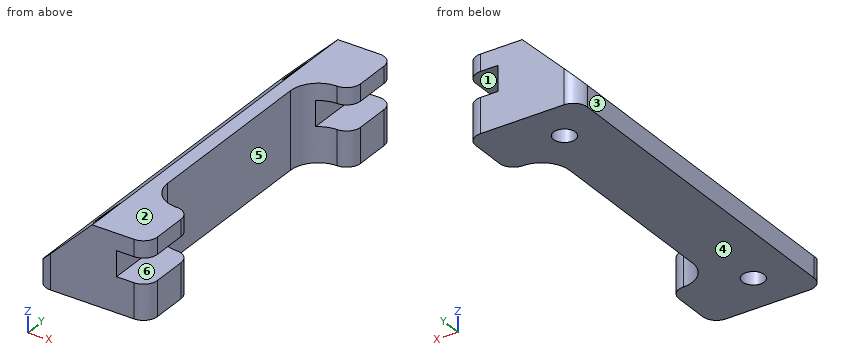
Autodesk Inventor part; units mm, degrees
ref_plane "YZ Plane" through (0, 0, 0) normal (1, 0, 0) x (0, 1, 0)
ref_plane "XZ Plane" through (0, 0, 0) normal (0, 1, 0) x (-1, 0, 0)
ref_plane "XY Plane" through (0, 0, 0) normal (0, 0, 1) x (1, 0, 0)
sketch "Sketch1" plane through (0, 0, 0) normal (0, 0, 1) x (1, 0, 0)
  line L0 (-4, 13) -> (-4, -13)
  line L1 (-4, -13) -> (4, -13)
  line L2 (4, -13) -> (4, 13)
  line L3 (4, 13) -> (-4, 13)
  line L4 (-1, -10) -> (-1, 10) construction
  circle A0 centre (-1, 10) radius 3 construction
  point P0 (0, 0)
  point P1 (0, 13)
  point P2 (-4, 0)
  point P3 (-1, 0)
  dimension "d0" = 26
  dimension "d2" = 20
  dimension "d5" = 5
extrude "Extrusion1" add sketch "Sketch1" along normal mid plane 5.5
sketch "Sketch2" plane through (0, 0, 2.75) normal (0, 0, 1) x (1, 0, 0)
  point P0 (0, 0)
  point P1 (-1, 10)
  point P2 (-1, -10)
hole "Hole1" at (-1, 10, 2.75) at (-1, -10, 2.75) direction (0, 0, -1) diameter 1.567 end through all
sketch "Sketch3" plane through (-4, -13, 2.75) normal (0, -1, 0) x (1, 0, 0)
  line L0 (8, -5.5) -> (8, 0)
  line L1 (0, 0) -> (8, 0)
  line L2 (0, -5.5) -> (0, 0)
  line L3 (8, -5.5) -> (0, -5.5)
  line L4 (8, -5.5) -> (8, 0)
  line L5 (8, -1.2) -> (5.75, -1.2)
  line L6 (5.75, -1.2) -> (5.75, -3)
  line L7 (5.75, -3) -> (8, -3)
  line L8 (8, -3) -> (8, -1.2)
  point P0 (4, -2.75)
  dimension "d13" = 2.5
  dimension "d14" = 1.8
  dimension "d15" = 2.25
extrude "Extrusion2" cut sketch "Sketch3" against normal through all contours L7 L6 L5 L0
chamfer "Chamfer1" distance 4 angle 45 1 edges at (-4, 0, 2.75)
sketch "Sketch4" plane through (0, 0, 2.75) normal (0, 0, 1) x (1, 0, 0)
  line L0 (0, -13) -> (0, 13)
  line L1 (0, -13) -> (4, -13)
  line L2 (4, -13) -> (4, 13)
  line L3 (4, 13) -> (0, 13)
  line L4 (4, 13) -> (4, -13)
  line L5 (4, 8.5) -> (1, 8.5)
  line L6 (1, 8.5) -> (1, -8.5)
  line L7 (1, -8.5) -> (4, -8.5)
  line L8 (4, -8.5) -> (4, 8.5)
  line L9 (4, -13) -> (4, 13)
  point P0 (0, 0)
  point P1 (4, 0)
  dimension "d21" = 3
  dimension "d22" = 17
extrude "Extrusion3" cut sketch "Sketch4" against normal through all contours L7 L6 L5 L2
fillet "Fillet1" radius 2 2 edges at (1, 8.5, 0) (1, -8.5, 0)
fillet "Fillet1" radius 1 10 edges at (4, -8.5, 2.15) (4, -13, 2.15) (4, -13, -1.5) (4, -8.5, -1.5) (4, 13, 2.15) (4, 8.5, 2.15) (4, 8.5, -1.5) (4, 13, -1.5) (-4, 13, -2) (-4, -13, -2)
properties part number "Payload_CameraSupport" material "Aluminum"
Source: CAD feature listing. Evaluate the final solid. Frame: model axes, mm. Face numbers are marked on the shaded views. A direction names the side the tool comes from. Give positions to 0.01 mm unless a question says otherwise; leave off trailing zeros. Write each loop counter-clockwise with the first axis right and the second up, starting at its lowest first coordinate (ties: lowest second). Pieces come first, ordered by that corner, then holes. Notation, with made-up numbers: (35.25, 51.25) - (93.25, 51.25) arc R16 ccw to (93.25, 68.25) - close; hole circle Ø7 at (76.5, 39.25). An arc over 180 degrees is marked (long way). One line per item, written item: value. Start each with the question number.
Q1. Section query B-B, the plane z = 0.35. Return the cut outline in (x, y), then the cut area to 3 significant figures.
Q2. Section query D-D, the plane x = 2.25. Return the cut outline in (y, z).
Q3. Section query C-C, the plane y = 10. Return the cut outline in (x, z), then the cut area to 3 significant figures.
Q4. Material intervals for probe 1 along Y at (x, z) = (-1, 0.2); probe 2 along Z at (x, y) = (2, -8.75); probe 3 along X at (y, z) = (-10, -1.5), sorted ascending. Write a range as from..to.
Q5. Section query A-A, the plane x = -1. Return the cut outline in (y, z).
Q6. Draft query along Z for the marked faces 1, 2 and 3. Return one class per face: +Z half, -Z half, draft (parallel to the pull), parting line (faces both ways), or undercut.
Q7. Set-up query: the marked faces 4, 5 and 6. Return all of +Z, -Z, +X, -X, +Y, -Y with unobstructed straight access to the full face (end or side cutting, diameter ignored); none if empty.
Q8. First-contact query: pin 1 Ø2 at (y, z) = (1, 1.5) entering from -X; pin 2 Ø2 at (x, y) = (-1, 10) entering from -Z; pin 3 Ø1.4 at (y, z) = (11.5, 0.5) entering from +X; pin 4 Ø2 at (x, y) = (3, 0) entering from +Z. Flat tips, straight axial feed; report the tip coordinate or a pass-through.
Answer:
1. outline: (-2.4, -13) - (1.75, -13) - (1.75, -8.06) arc R2 cw to (1, -6.5) - (1, 6.5) arc R2 cw to (1.75, 8.06) - (1.75, 13) - (-2.4, 13) - close; hole circle Ø1.57 at (-1, -10); hole circle Ø1.57 at (-1, 10)
1. area: 92.7 mm2
2. outline: (-13, -2.75) - (-8.35, -2.75) - (-8.35, -0.25) - (-13, -0.25) - close; (-13, 1.55) - (-8.35, 1.55) - (-8.35, 2.75) - (-13, 2.75) - close; (8.35, -2.75) - (13, -2.75) - (13, -0.25) - (8.35, -0.25) - close; (8.35, 1.55) - (13, 1.55) - (13, 2.75) - (8.35, 2.75) - close
3. outline: (-4, -2.75) - (-1.78, -2.75) - (-1.78, 0.97) - (-4, -1.25) - close; (-0.22, -2.75) - (4, -2.75) - (4, -0.25) - (1.75, -0.25) - (1.75, 1.55) - (4, 1.55) - (4, 2.75) - (0, 2.75) - (-0.22, 2.53) - close
3. area: 24.9 mm2
4. probe 1: y = -13..-10.78, -9.22..9.22, 10.78..13
4. probe 2: z = -2.75..-0.25, 1.55..2.75
4. probe 3: x = -4..-1.78, -0.22..4
5. outline: (-13, -2.75) - (-10.78, -2.75) - (-10.78, 1.75) - (-13, 1.75) - close; (-9.22, -2.75) - (9.22, -2.75) - (9.22, 1.75) - (-9.22, 1.75) - close; (10.78, -2.75) - (13, -2.75) - (13, 1.75) - (10.78, 1.75) - close
6. face 1: undercut
6. face 2: +Z half
6. face 3: draft
7. face 4: -Z, +X, -X, +Y, -Y
7. face 5: +Z, -Z, +X
7. face 6: +X, +Y, -Y
8. pin 1: stops at x = -2.25
8. pin 2: stops at z = -2.75
8. pin 3: stops at x = 1.75
8. pin 4: passes through
